from build123d import *

# Parameters (mm, degrees)
F0_W     = 99.2823541164
F0_H     = 20.0983081013
F1_DEPTH = 20.32
F3_D     = 10.16
F5_D     = 10.16
F7_D     = 7.62


with BuildPart() as f1:
    # F0 (on Front) → F1 (new body)
    with BuildSketch(Plane.XZ):
        with Locations((49.6411770582, -10.0491540506)):
            Rectangle(F0_W, F0_H)
    extrude(amount=F1_DEPTH)

    # F3 (through all)
    with Locations(Plane(origin=(0, 0, 0), x_dir=(1, 0, 0), z_dir=(0, 1, 0))):
        with Locations((10.5173690245, 8.8591091335)):
            Hole(F3_D / 2)

    # F5 (through all)
    with Locations(Plane.XZ.offset(20.32)):
        with Locations((88.3474946022, -9.0083088726)):
            Hole(F5_D / 2)

    # F7 (through all)
    with Locations(Plane.XZ.offset(20.32)):
        with Locations((27.3221246898, -9.2888381332), (74.1779506207, -9.2888381332)):
            Hole(F7_D / 2)


solid = f1.part
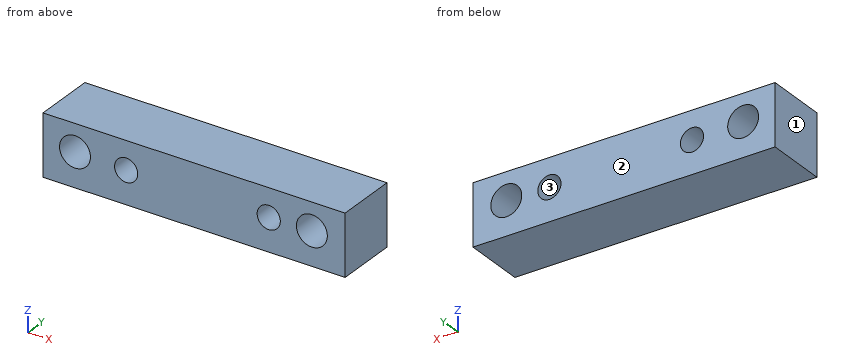
Build history of the part. All positions in model axes, mm. Face numbers are marked on the shaded views. Coordinates: 2 decimals unless noted, no trailing zeros. Order: outer loops, then holes, each group sorted by start corner. A loop starts at its lowest first (then second) coordinate and runs counter-clockwise, first axis right, second up. Notation, with made-up numbers: (29.5, -25.75) -> (61.5, -25.75) arc R17 cw to (61.5, 0.25) -> close; hole circle Ø6 at (28.5, -32). An arc over 180 degrees is marked (long way). One line per item, written item: value.
(1) Slice it at B-B, the plane x = 85. List the corners of the cut face in (y, z).
Checked values:
outline: (-20.32, -20.1) -> (0, -20.1) -> (0, -12.83) -> (-20.32, -12.83) -> close; (-20.32, -5.19) -> (0, -5.19) -> (0, 0) -> (-20.32, 0) -> close
(2) Slice it at C-C, the plane y = -13. List the corners of the cut face in (x, z).
Checked values:
outline: (0, -20.1) -> (99.28, -20.1) -> (99.28, 0) -> (0, 0) -> close; hole circle Ø10.16 at (10.52, -8.86); hole circle Ø7.62 at (27.32, -9.29); hole circle Ø7.62 at (74.18, -9.29); hole circle Ø10.16 at (88.35, -9.01)
(3) Mould opens along X. For the marked faces 1, 2 and 3 say: pulls with the +X half, pulls with the -X half, needs draft (parallel to the pull), parting line crosses it, or undercut.
Checked values:
face 1: pulls with the -X half
face 2: needs draft
face 3: undercut
(4) Probe line 1 (X direction, y = -13, z = -9.75); line 2 (X direction, y = -9.5, z = -12.25); line 3 (X direction, y = -5.25, z = -13.5). List the from-to ranges inside material, lowest first. Write a range as [from, to].
Checked values:
line 1: [0, 5.52], [15.52, 23.54], [31.1, 70.4], [77.96, 83.32], [93.37, 99.28]
line 2: [0, 6.73], [14.3, 24.92], [29.72, 71.78], [76.58, 84.44], [92.26, 99.28]
line 3: [0, 8.45], [12.58, 85.97], [90.72, 99.28]
(5) Slice it at A-A, the plane z = -10.75. List the corners of the cut face in (x, y).
Checked values:
outline: (0, -20.32) -> (5.8, -20.32) -> (5.8, 0) -> (0, 0) -> close; (15.23, -20.32) -> (23.8, -20.32) -> (23.8, 0) -> (15.23, 0) -> close; (30.84, -20.32) -> (70.66, -20.32) -> (70.66, 0) -> (30.84, 0) -> close; (77.7, -20.32) -> (83.58, -20.32) -> (83.58, 0) -> (77.7, 0) -> close; (93.12, -20.32) -> (99.28, -20.32) -> (99.28, 0) -> (93.12, 0) -> close
